Print and shaded views of the part. All mm, measured from the part's lowest x, y and z. A direction names the side the tool comes from. Round coordinates to 2 decimals unless told otherwise and drop trailing zeros. Write each loop counter-clockwise with the first axis right and the second up, starting at its lowest first coordinate (ties: lowest second). Pieces come first, ordered by that corner, then holes. Notation, with made-up numbers: M -24,-29.75 L -6,-29.75 A20 cw -6,-6.75 Z; hole C -30,14 d1. An arc over 180 degrees is marked long. Write item = value, one per line. Start each with the question number.
Q1. Band-saw the part on A-A on z = 12. State how many separate pieces and enclosed holes the cut face has, plus the area to 3 significant figures.
Q2. Tool access for the marked faces 3 and 4: list every direction of +Z, -Z, +X, -X, +Y, -Y with a clear straight run to the whole face (end or side of a thin tool).
Q3. Band-saw the part on B-B on y = 12. Write the cut outline in (x, z) (1 decimal), plus the area to 3 significant figures.
Q4. Band-saw the part on C-C on x = 30.5. Write the cut outline in (y, z).
Q5. Drop flat-ended pins along their axis: P1, Ø6, axis at x = 5.5, y = 19, coming from the +Z side; P2, Ø3, axis at x = 26, z = 15.5, coming from the -Y side; P3, Ø3, axis at x = 4.5, z = 15.5, coming from the -Y side. Give the stop position or say it passes through.
Q6. Band-saw the part on D-D on x = 19. Write the cut outline in (y, z).
Q7. Pull direction Z, two halves, no side cores. Call the marked faces 1 and 2: released by +Z, released by -Z, zero draft, split by the parting line, or undercut.
Q8. Probe L1, parallel to Z at x = 25, y = 12; L2, parallel to Z at x = 28.5, y = 18.75 (1 decimal); L3, parallel to X at y = 1.55, z = 12. List the from-to ranges inside material, lowest first.
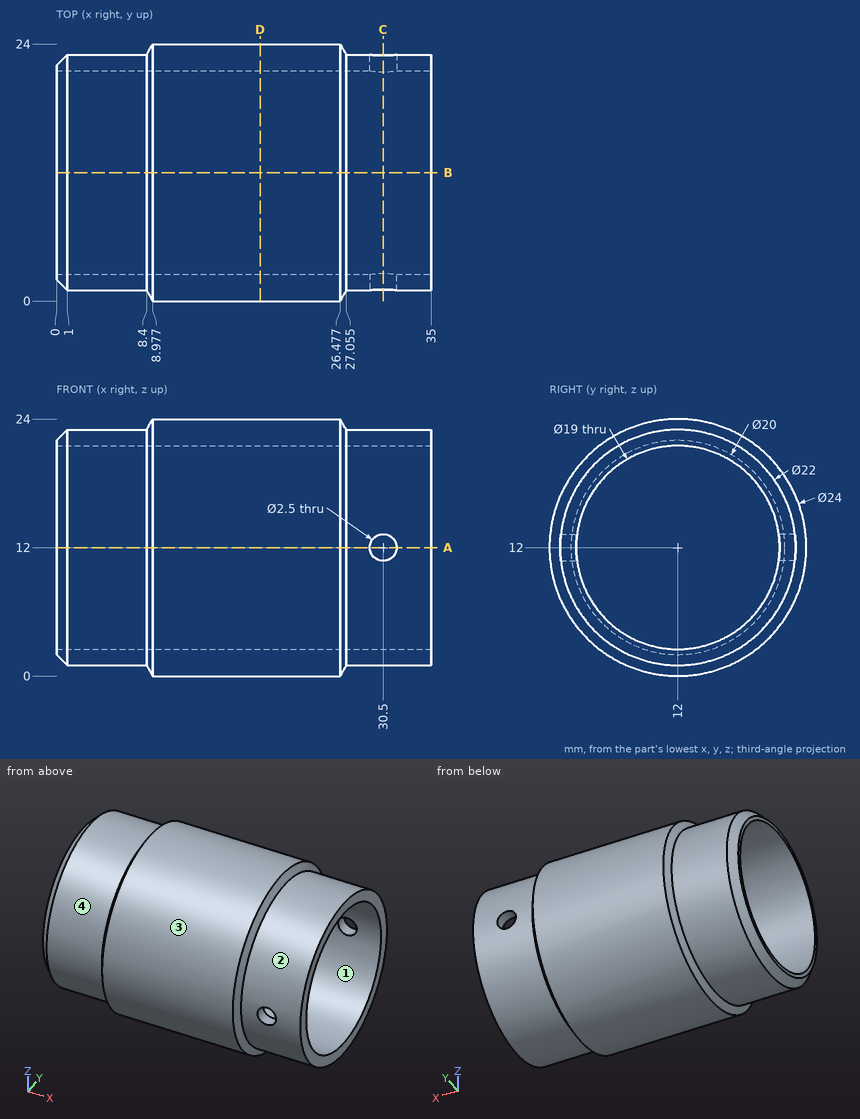
Conclusion:
q1.separate_pieces = 4
q1.enclosed_holes = 0
q1.area = 133 mm^2
q2.face_3 = +X, -X
q2.face_4 = -X
q3.outline = M 0,2 L 1,1 L 8.4,1 L 9,0 L 26.5,0 L 27.1,1 L 35,1 L 35,2.5 L 0,2.5 Z; M 0,21.5 L 35,21.5 L 35,23 L 27.1,23 L 26.5,24 L 9,24 L 8.4,23 L 1,23 L 0,22 Z
q3.area = 140 mm^2
q4.outline = M 1.07,10.75 A11 ccw 22.93,10.75 L 21.42,10.75 A9.5 cw 2.58,10.75 Z; M 1.07,13.25 L 2.58,13.25 A9.5 cw 21.42,13.25 L 22.93,13.25 A11 ccw Z
q5.P1 = 22.25
q5.P2 = 0.17
q5.P3 = 1.18
q6.outline = C 12,12 d24; hole C 12,12 d19
q7.face_1 = undercut
q7.face_2 = split by the parting line
q8.L1 = 0 to 2.5, 21.5 to 24
q8.L2 = 3.3 to 5.3, 18.7 to 20.7
q8.L3 = 0.45 to 29.25, 31.75 to 35
